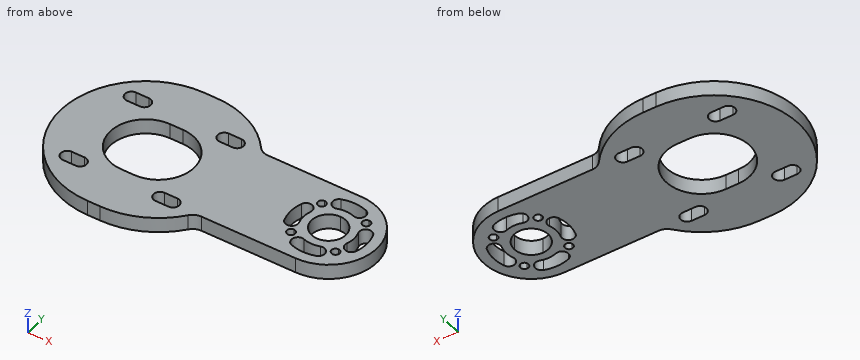
```python
from build123d import *

# Parameters (mm, degrees)
F1_DEPTH = 6
F3_DEPTH = 25


with BuildPart() as f1:
    # F0 (on Top) → F1 (new body)
    with BuildSketch(Plane.XY):
        with BuildLine():
            Line((32.653986447, -19), (70, -19))
            ThreePointArc((70, -19), (89, 0), (70, 19))
            Line((70, 19), (32.653986447, 19))
            ThreePointArc((32.653986447, 19), (30.4842417137, 19.4953126865), (28.7443778175, 20.8831168831))
            ThreePointArc((28.7443778175, 20.8831168831), (17.0872897133, 30.1814050003), (2.55, 33.5))
            Line((2.55, 33.5), (-2.55, 33.5))
            ThreePointArc((-2.55, 33.5), (-36.05, 0), (-2.55, -33.5))
            Line((-2.55, -33.5), (2.55, -33.5))
            ThreePointArc((2.55, -33.5), (17.0872897133, -30.1814050003), (28.7443778175, -20.8831168831))
            ThreePointArc((28.7443778175, -20.8831168831), (30.4842417137, -19.4953126865), (32.653986447, -19))
        make_face()
        with BuildLine():
            Line((-15.8347763109, -20.9347763109), (-20.9347763109, -20.9347763109))
            ThreePointArc((-20.9347763109, -20.9347763109), (-23.4847763109, -18.3847763109), (-20.9347763109, -15.8347763109))
            Line((-20.9347763109, -15.8347763109), (-15.8347763109, -15.8347763109))
            ThreePointArc((-15.8347763109, -15.8347763109), (-13.2847763109, -18.3847763109), (-15.8347763109, -20.9347763109))
        make_face(mode=Mode.SUBTRACT)
        with BuildLine():
            Line((20.9347763109, -20.9347763109), (15.8347763109, -20.9347763109))
            ThreePointArc((15.8347763109, -20.9347763109), (13.2847763109, -18.3847763109), (15.8347763109, -15.8347763109))
            Line((15.8347763109, -15.8347763109), (20.9347763109, -15.8347763109))
            ThreePointArc((20.9347763109, -15.8347763109), (23.4847763109, -18.3847763109), (20.9347763109, -20.9347763109))
        make_face(mode=Mode.SUBTRACT)
        with BuildLine():
            ThreePointArc((61.1611652352, -7.2388347648), (62.2925360851, -7.7074639149), (62.7611652352, -8.8388347648))
            ThreePointArc((62.7611652352, -8.8388347648), (62.2925360851, -9.9702056147), (61.1611652352, -10.4388347648))
            ThreePointArc((61.1611652352, -10.4388347648), (59.5611652352, -8.8388347648), (61.1611652352, -7.2388347648))
        make_face(mode=Mode.SUBTRACT)
        with BuildLine():
            ThreePointArc((78.8388347648, -7.2388347648), (79.9702056147, -7.7074639149), (80.4388347648, -8.8388347648))
            ThreePointArc((80.4388347648, -8.8388347648), (79.9702056147, -9.9702056147), (78.8388347648, -10.4388347648))
            ThreePointArc((78.8388347648, -10.4388347648), (77.2388347648, -8.8388347648), (78.8388347648, -7.2388347648))
        make_face(mode=Mode.SUBTRACT)
        with BuildLine():
            Line((-2.55, 14), (2.55, 14))
            ThreePointArc((2.55, 14), (16.55, 0), (2.55, -14))
            Line((2.55, -14), (-2.55, -14))
            ThreePointArc((-2.55, -14), (-16.55, 0), (-2.55, 14))
        make_face(mode=Mode.SUBTRACT)
        with BuildLine():
            Line((-15.8347763109, 15.8347763109), (-20.9347763109, 15.8347763109))
            ThreePointArc((-20.9347763109, 15.8347763109), (-23.4847763109, 18.3847763109), (-20.9347763109, 20.9347763109))
            Line((-20.9347763109, 20.9347763109), (-15.8347763109, 20.9347763109))
            ThreePointArc((-15.8347763109, 20.9347763109), (-13.2847763109, 18.3847763109), (-15.8347763109, 15.8347763109))
        make_face(mode=Mode.SUBTRACT)
        with BuildLine():
            Line((20.9347763109, 15.8347763109), (15.8347763109, 15.8347763109))
            ThreePointArc((15.8347763109, 15.8347763109), (13.2847763109, 18.3847763109), (15.8347763109, 20.9347763109))
            Line((15.8347763109, 20.9347763109), (20.9347763109, 20.9347763109))
            ThreePointArc((20.9347763109, 20.9347763109), (23.4847763109, 18.3847763109), (20.9347763109, 15.8347763109))
        make_face(mode=Mode.SUBTRACT)
        with BuildLine():
            ThreePointArc((70, 6.75), (74.772970773, 4.772970773), (76.75, 0))
            ThreePointArc((76.75, 0), (74.772970773, -4.772970773), (70, -6.75))
            ThreePointArc((70, -6.75), (63.25, 0), (70, 6.75))
        make_face(mode=Mode.SUBTRACT)
        with BuildLine():
            ThreePointArc((61.1611652352, 10.4388347648), (62.2925360851, 9.9702056147), (62.7611652352, 8.8388347648))
            ThreePointArc((62.7611652352, 8.8388347648), (62.2925360851, 7.7074639149), (61.1611652352, 7.2388347648))
            ThreePointArc((61.1611652352, 7.2388347648), (59.5611652352, 8.8388347648), (61.1611652352, 10.4388347648))
        make_face(mode=Mode.SUBTRACT)
        with BuildLine():
            ThreePointArc((78.8388347648, 10.4388347648), (79.9702056147, 9.9702056147), (80.4388347648, 8.8388347648))
            ThreePointArc((80.4388347648, 8.8388347648), (79.9702056147, 7.7074639149), (78.8388347648, 7.2388347648))
            ThreePointArc((78.8388347648, 7.2388347648), (77.2388347648, 8.8388347648), (78.8388347648, 10.4388347648))
        make_face(mode=Mode.SUBTRACT)
    extrude(amount=F1_DEPTH)

    # F2 (on face) → F3 (cut)
    with BuildSketch(Plane.XY.offset(6)):
        with BuildLine():
            ThreePointArc((60.544814244, 3.2556815446), (58.9949381912, 6.4333983697), (55.817221366, 4.8835223169))
            ThreePointArc((55.817221366, 4.8835223169), (55, 0), (55.817221366, -4.8835223169))
            ThreePointArc((55.817221366, -4.8835223169), (58.9949381912, -6.4333983697), (60.544814244, -3.2556815446))
            ThreePointArc((60.544814244, -3.2556815446), (60, 0), (60.544814244, 3.2556815446))
        make_face()
        with BuildLine():
            ThreePointArc((66.7443184554, -9.455185756), (63.5666016303, -11.0050618088), (65.1164776831, -14.182778634))
            ThreePointArc((65.1164776831, -14.182778634), (70, -15), (74.8835223169, -14.182778634))
            ThreePointArc((74.8835223169, -14.182778634), (76.4333983697, -11.0050618088), (73.2556815446, -9.455185756))
            ThreePointArc((73.2556815446, -9.455185756), (70, -10), (66.7443184554, -9.455185756))
        make_face()
        with BuildLine():
            ThreePointArc((79.455185756, -3.2556815446), (81.0050618088, -6.4333983697), (84.182778634, -4.8835223169))
            ThreePointArc((84.182778634, -4.8835223169), (85, 0), (84.182778634, 4.8835223169))
            ThreePointArc((84.182778634, 4.8835223169), (81.0050618088, 6.4333983697), (79.455185756, 3.2556815446))
            ThreePointArc((79.455185756, 3.2556815446), (80, 0), (79.455185756, -3.2556815446))
        make_face()
        with BuildLine():
            ThreePointArc((73.2556815446, 9.455185756), (76.4333983697, 11.0050618088), (74.8835223169, 14.182778634))
            ThreePointArc((74.8835223169, 14.182778634), (70, 15), (65.1164776831, 14.182778634))
            ThreePointArc((65.1164776831, 14.182778634), (63.5666016303, 11.0050618088), (66.7443184554, 9.455185756))
            ThreePointArc((66.7443184554, 9.455185756), (70, 10), (73.2556815446, 9.455185756))
        make_face()
    extrude(amount=-F3_DEPTH, mode=Mode.SUBTRACT)


solid = f1.part
```
CAD build for the part. Positions are in the model's coordinates, mm. Round coordinates to 2 decimals unless told otherwise and drop trailing zeros. Write each loop counter-clockwise with the first axis right and the second up, starting at its lowest first coordinate (ties: lowest second). Pieces come first, ordered by that corner, then holes. Notation, with made-up numbers: (88.5, 82) - (119.5, 82) arc R15 ccw to (119.5, 107) - close; hole circle Ø4 at (24.25, 33). An arc over 180 degrees is marked (long way). Write item = value, one per line. Start each with the question number.
Q1. Probe L1, parallel to Y at x = 79, z = 4.5; L2, parallel to Y at x = 66, z = 1; L3, parallel to X at y = 3, z = 1.15. List the from-to ranges inside material, lowest first. Write a range as from..to.
Q2. Band-saw the part on B-B (y = -12). Give the cut face in (x, z).
Q3. Band-saw the part on C-C (z = 3.2). Count the separate pieces of the cut face and the enclosed holes in it, then the cut area to 3 significant figures.
Q4. Band-saw the part on D-D (x = 25). Give the cut face in (y, z).
Q5. Band-saw the part on A-A (x = 58). Give the cut face in (y, z), then the cut area to 3 significant figures.
Q6. Drop flat-ended pins along their axis: pin 1 (2.5 mm diameter, centred on x = -17.5, z = 2.5, fed in from +Y); pin 2 (1.5 mm diameter, centred on x = 19.5, z = 4.5, fed in from +Y); pin 3 (3 mm diameter, centred on x = 65, z = 2, fed in from -Y). Give the stop position or say it passes through.
Answers below:
q1.L1 = -16.73..-10.43, -7.25..7.25, 10.43..16.73
q1.L2 = -19..-14.46, -9.32..-5.44, 5.44..9.32, 14.46..19
q1.L3 = -35.92..-16.22, 16.22..55.3, 60.46..63.95, 76.05..79.54, 84.7..88.76
q2.outline = (-33.83, 0) - (-9.76, 0) - (-9.76, 6) - (-33.83, 6) - close; (9.76, 0) - (63.44, 0) - (63.44, 6) - (9.76, 6) - close; (76.56, 0) - (84.73, 0) - (84.73, 6) - (76.56, 6) - close
q3.separate_pieces = 1
q3.enclosed_holes = 14
q3.area = 4,430 mm2
q4.outline = (-24.86, 0) - (24.86, 0) - (24.86, 6) - (-24.86, 6) - close
q5.outline = (-19, 0) - (-6.56, 0) - (-6.56, 6) - (-19, 6) - close; (6.56, 0) - (19, 0) - (19, 6) - (6.56, 6) - close
q5.area = 149 mm2
q6.pin_1 = 30.57
q6.pin_2 = 29.32
q6.pin_3 = -19
